Input: part model. Units: mm. Frame: model coordinates. A direction names the side the tool comes from. Round coordinates to 2 decimals unless told otherwise and drop trailing zeros. Order: outer loops, then holes, each group sorted by start corner. A loop starts at its lowest first (then second) coordinate and runs counter-clockwise, first axis right, second up. Notation, with made-up numbers: (62, 15.25) -> (83, 15.25) arc R26 ccw to (83, 29.25) -> close; hole circle Ø2 at (57, 79.25). An arc over 180 degrees is marked (long way). Use a Markdown table: item, result.
from build123d import *

# Parameters (mm, degrees)
ESQUISSE1_R                                    = 3.15
BOSS_EXTRU_1_DEPTH                             = 19
ESQUISSE2_W                                    = 9
ESQUISSE2_H                                    = 12.5
ENL_V_MAT_EXTRU_1_DEPTH                        = 15
FRAISAGE_POUR_VIS_T_TE_FRAIS_E_M31_D           = 3.4
FRAISAGE_POUR_VIS_T_TE_FRAIS_E_M31_CSINK_D     = 6.3
FRAISAGE_POUR_VIS_T_TE_FRAIS_E_M31_CSINK_ANGLE = 90
CONG_1_R                                       = 2.5
CONG_2_R                                       = 0.5


with BuildPart() as part:
    # Esquisse1 → Boss.-Extru.1 (new body)
    with BuildSketch(Plane.XY):
        with BuildLine():
            Line((-5.5, 3.5), (-5.5, 14))
            ThreePointArc((-5.5, 14), (0, 19.5), (5.5, 14))
            Line((5.5, 14), (5.5, 3.5))
            Line((5.5, 3.5), (-5.5, 3.5))
        make_face()
        with Locations((0, 14)):
            Circle(ESQUISSE1_R, mode=Mode.SUBTRACT)
    extrude(amount=BOSS_EXTRU_1_DEPTH)

    # Esquisse2 → Enlèv. mat.-Extru.1 (cut)
    with BuildSketch(Plane(origin=(5.5, 0, 0), x_dir=(0, 0, -1), z_dir=(1, 0, 0))):
        with Locations((-9.5, 13.25)):
            Rectangle(ESQUISSE2_W, ESQUISSE2_H)
    extrude(amount=-ENL_V_MAT_EXTRU_1_DEPTH, mode=Mode.SUBTRACT)

    # Fraisage pour vis à tête fraisée M31 (through all)
    with Locations(Plane(origin=(0, 7, 0), x_dir=(1, 0, 0), z_dir=(0, 1, 0))):
        with Locations((0, -9.5)):
            CounterSinkHole(FRAISAGE_POUR_VIS_T_TE_FRAIS_E_M31_D / 2, FRAISAGE_POUR_VIS_T_TE_FRAIS_E_M31_CSINK_D / 2, counter_sink_angle=FRAISAGE_POUR_VIS_T_TE_FRAIS_E_M31_CSINK_ANGLE)

    # Congé1
    cong_1_edges = [part.edges().sort_by_distance(p)[0] for p in [
        (5.5, 8.75, 0),
        (5.5, 8.75, 19),
        (-5.5, 8.75, 19),
        (-5.5, 8.75, 0),
    ]]
    fillet(cong_1_edges, radius=CONG_1_R)

    # Congé2
    cong_2_edges = [part.edges().sort_by_distance(p)[0] for p in [
        (0, 7, 14),
        (0, 7, 5),
    ]]
    fillet(cong_2_edges, radius=CONG_2_R)


solid = part.part
1) Cut plane A-A on z = 9.5. Return loops of the section in (x, y).
Answer key:
| item | result |
|---|---|
| outline | (-5.5, 3.5) -> (-1.7, 3.5) -> (-1.7, 5.55) -> (-3.15, 7) -> (-5.5, 7) -> close; (1.7, 3.5) -> (5.5, 3.5) -> (5.5, 7) -> (3.15, 7) -> (1.7, 5.55) -> close |
2) Cut plane C-C on y = 8.5. Return loops of the section in (x, z).
Answer key:
| item | result |
|---|---|
| outline | (-5.5, 2.5) arc R2.5 ccw to (-3, 0) -> (3, 0) arc R2.5 ccw to (5.5, 2.5) -> (5.5, 5) -> (-5.5, 5) -> close; (-5.5, 14) -> (5.5, 14) -> (5.5, 16.5) arc R2.5 ccw to (3, 19) -> (-3, 19) arc R2.5 ccw to (-5.5, 16.5) -> close |
3) Set-up query: faces 1 (the face through (-2.5, 12.083, 16.465)), 2 (the face through (0.1, 10.7, 14)). Return all of +Z, -Z, +X, -X, +Y, -Y with unobstructed straight access to the full face (end or side cutting, diameter ignored); none if empty.
Answer key:
| item | result |
|---|---|
| face 1 | +Z, -Z |
| face 2 | +X, -X, +Y |
4) Cut plane D-D on x = -0.5. State how many separate pieces and enclosed holes the cut face has, and give its area (3 significant figures).
Answer key:
| item | result |
|---|---|
| separate pieces | 4 |
| enclosed holes | 0 |
| area | 113 mm^2 |
5) Ray query, probe 1 along X at (y, z) = (4.6, 9.5); probe 2 along X at (y, z) = (14, 2.95); probe 3 along Z at (x, y) = (-1, 10). Return the intervals inside material, ascending.
Answer key:
| item | result |
|---|---|
| probe 1 | x = -5.5 to -1.7, 1.7 to 5.5 |
| probe 2 | x = -5.5 to -3.15, 3.15 to 5.5 |
| probe 3 | z = 0 to 5, 14 to 19 |
6) Cut plane B-B on y = 6. Return loops of the section in (x, z), and give its area (3 significant figures).
Answer key:
| item | result |
|---|---|
| outline | (-5.5, 2.5) arc R2.5 ccw to (-3, 0) -> (3, 0) arc R2.5 ccw to (5.5, 2.5) -> (5.5, 16.5) arc R2.5 ccw to (3, 19) -> (-3, 19) arc R2.5 ccw to (-5.5, 16.5) -> close; hole circle Ø4.3 at (0, 9.5) |
| area | 189 mm^2 |
7) Draft query along X for faces 3 (the face through (0, 7, 13)), 4 (the face through (0.37, 4.51, 11.16)), 5 (the face through (5, 8, 1)). Return one class per face: released by +X, released by -X, zero draft, split by the parting line, or undercut.
Answer key:
| item | result |
|---|---|
| face 3 | zero draft |
| face 4 | undercut |
| face 5 | released by +X |
8) Contact query for flat-ended pins moving along their axis: P1, Ø1, axis at x = 1, y = 13.5, coming from the +Z side; P2, Ø2.5, axis at x = -0.5, z = 8.5, coming from the +Y side; P3, Ø2, axis at x = -2, z = 12, coming from the +Y side. Output: stop coordinate, or through.
Answer key:
| item | result |
|---|---|
| P1 | passes through |
| P2 | stops at y = 6.22 |
| P3 | stops at y = 7 |
